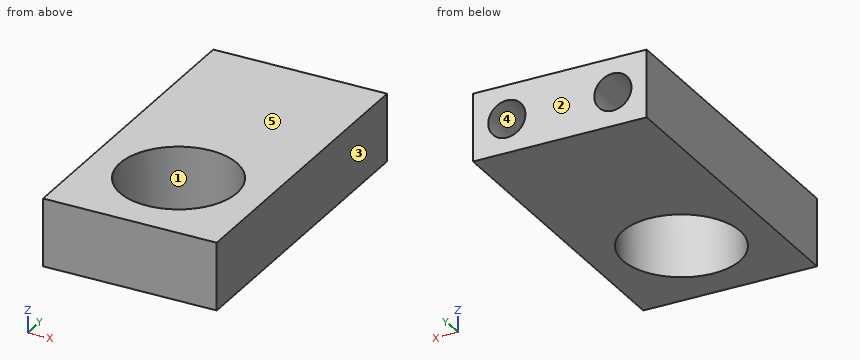
from build123d import *

# Parameters (mm, degrees)
SKETCH1_W                                     = 15.4
SKETCH1_H                                     = 6
BOSS_EXTRUDE1_DEPTH                           = 28
TAP_DRILL_FOR_M4X0_7_TAP1_D                   = 3.3
TAP_DRILL_FOR_M4X0_7_TAP1_DEPTH               = 13.4
TAP_DRILL_FOR_M4X0_7_TAP1_TIP                 = 0.991420021
CUT_EXTRUDE_PRESS_FIT_HOLE_FOR_SOLENOID_REACH = 31.653
SKETCH4_R                                     = 5.2


with BuildPart() as part:
    # Sketch1 → Boss-Extrude1 (new body)
    with BuildSketch(Plane(origin=(0, 0, 0), x_dir=(1, 0, 0), z_dir=(0, 1, 0))):
        Rectangle(SKETCH1_W, SKETCH1_H)
    extrude(amount=BOSS_EXTRUDE1_DEPTH)

    # Tap Drill for M4x0.7 Tap1
    with Locations(Plane(origin=(-4.7, 28, 0), x_dir=(0, 0, 1), z_dir=(0, 1, 0))):
        with Locations((0, 0), (0, 9.4)):
            Hole(TAP_DRILL_FOR_M4X0_7_TAP1_D / 2, depth=TAP_DRILL_FOR_M4X0_7_TAP1_DEPTH)
            with Locations((0, 0, -(TAP_DRILL_FOR_M4X0_7_TAP1_DEPTH + TAP_DRILL_FOR_M4X0_7_TAP1_TIP / 2))):  # 118° drill point
                Cone(0, TAP_DRILL_FOR_M4X0_7_TAP1_D / 2, TAP_DRILL_FOR_M4X0_7_TAP1_TIP, mode=Mode.SUBTRACT)

    # Sketch4 → Cut-Extrude Press Fit hole for solenoid tube (cut, up to next)
    with BuildSketch(Plane.XY.offset(3), mode=Mode.PRIVATE) as cut_extrude_press_fit_hole_for_solenoid_sk1:
        with Locations((0, 8)):
            Circle(SKETCH4_R)
    cut_extrude_press_fit_hole_for_solenoid_tool1 = extrude(cut_extrude_press_fit_hole_for_solenoid_sk1.sketch, amount=-CUT_EXTRUDE_PRESS_FIT_HOLE_FOR_SOLENOID_REACH, mode=Mode.PRIVATE) & part.part
    add(cut_extrude_press_fit_hole_for_solenoid_tool1.solids().sort_by_distance((0, 8, 3))[0], mode=Mode.SUBTRACT)


solid = part.part
For this review, take the finished solid that the model builds, in its own axes (mm). Face numbers are marked on the shaded views. A direction names the side the tool comes from. Give positions to 0.01 mm unless a question says otherwise; leave off trailing zeros. Write each loop counter-clockwise with the first axis right and the second up, starting at its lowest first coordinate (ties: lowest second). Pieces come first, ordered by that corner, then holes. Notation, with made-up numbers: (13.25, 23) -> (62.25, 23) arc R35 ccw to (62.25, 61) -> close; hole circle Ø11 at (88.25, 70). An arc over 180 degrees is marked (long way). Use CSV: the item, a comma, the result in double quotes.
Q1. Tool access review of the marked faces 4 and 5: name each direction out of +Z, -Z, +X, -X, +Y, -Y from which nothing blocks a thin tool from reaching the whole face with its end or side.
Conclusion:
face 4,"+Y"
face 5,"+Z, +X, -X, +Y, -Y"
Q2. Take a section at B-B, the plane x = 0. Write out the cut boundary in (y, z).
Conclusion:
outline,"(0, -3) -> (2.8, -3) -> (2.8, 3) -> (0, 3) -> close; (13.2, -3) -> (28, -3) -> (28, 3) -> (13.2, 3) -> close"
Q3. Take a section at A-A, the plane y = 8. Write out the cut boundary in (x, z), then the cut area to 3 significant figures.
Conclusion:
outline,"(-7.7, -3) -> (-5.2, -3) -> (-5.2, 3) -> (-7.7, 3) -> close; (5.2, -3) -> (7.7, -3) -> (7.7, 3) -> (5.2, 3) -> close"
area,"30.0 mm2"
Q4. To check wall thickness, follow probe 1 along X at (y, z) = (18, 0); probe 2 along Z at (x, y) = (-4.7, 21.25); probe 3 along Y at (x, z) = (-0.25, 1.95). State the ranges of each line that lie inside material, in increasing order. Write a range as [from, to].
Conclusion:
probe 1,"[-7.7, -6.35], [-3.05, 3.05], [6.35, 7.7]"
probe 2,"[-3, -1.65], [1.65, 3]"
probe 3,"[0, 2.81], [13.19, 28]"
Q5. For P1, Ø2, axis at x = -4.7, z = 0, coming from the +Y side; P2, Ø3, axis at x = 4.7, z = 0, coming from the +Y side, all flat-tipped, find the tip position at first contact; note any pin that passes through.
Conclusion:
P1,"y = 14.21"
P2,"y = 14.51"
Q6. Take a section at D-D, the plane y = 25.5. Write out the cut boundary in (x, z).
Conclusion:
outline,"(-7.7, -3) -> (7.7, -3) -> (7.7, 3) -> (-7.7, 3) -> close; hole circle Ø3.3 at (-4.7, 0); hole circle Ø3.3 at (4.7, 0)"
Q7. Mouldability with a two-part tool opening along X and no side actions: class the marked faces 1, 2 and 3 as pulls with the +X half, pulls with the -X half, needs draft (parallel to the pull), parting line crosses it, or undercut.
Conclusion:
face 1,"undercut"
face 2,"needs draft"
face 3,"pulls with the +X half"
Q8. Take a section at C-C, the plane z = -2.4. Write out the cut boundary in (x, y).
Conclusion:
outline,"(-7.7, 0) -> (7.7, 0) -> (7.7, 28) -> (-7.7, 28) -> close; hole circle Ø10.4 at (0, 8)"
